from build123d import *

# Parameters (mm, degrees)
SKETCH1_R           = 4
BOSS_EXTRUDE1_DEPTH = 5
BOSS_EXTRUDE1_TAPER = 13
SKETCH2_R           = 4
BOSS_EXTRUDE2_DEPTH = 5
BOSS_EXTRUDE2_TAPER = 13
SKETCH3_R           = 4
BOSS_EXTRUDE3_DEPTH = 5
BOSS_EXTRUDE3_TAPER = 13
SKETCH4_R           = 2.85
BOSS_EXTRUDE4_DEPTH = 2
SKETCH5_R           = 2.85
BOSS_EXTRUDE5_DEPTH = 3
BOSS_EXTRUDE5_DRAFT = -35
SKETCH6_R           = 4.950622615
BOSS_EXTRUDE6_DEPTH = 15
BOSS_EXTRUDE6_TAPER = 12
SKETCH9_R           = 2
CUT_EXTRUDE1_DEPTH  = 20


with BuildPart() as part:
    # Sketch1 → Boss-Extrude1 (new body)
    with BuildSketch(Plane(origin=(0, 0, 0), x_dir=(0, 0, -1), z_dir=(1, 0, 0))):
        Circle(SKETCH1_R)
    extrude(amount=BOSS_EXTRUDE1_DEPTH, taper=BOSS_EXTRUDE1_TAPER)

    # Sketch2 → Boss-Extrude2 (add)
    with BuildSketch(Plane(origin=(5, 0, 0), x_dir=(0, 0, -1), z_dir=(1, 0, 0))):
        Circle(SKETCH2_R)
    extrude(amount=BOSS_EXTRUDE2_DEPTH, taper=BOSS_EXTRUDE2_TAPER)

    # Sketch3 → Boss-Extrude3 (add)
    with BuildSketch(Plane(origin=(10, 0, 0), x_dir=(0, 0, -1), z_dir=(1, 0, 0))):
        Circle(SKETCH3_R)
    extrude(amount=BOSS_EXTRUDE3_DEPTH, taper=BOSS_EXTRUDE3_TAPER)

    # Sketch4 → Boss-Extrude4 (add)
    with BuildSketch(Plane.ZY):
        Circle(SKETCH4_R)
    extrude(amount=BOSS_EXTRUDE4_DEPTH)


with BuildPart() as boss_extrude5_tool:
    # Sketch5 → Boss-Extrude5 (with draft: the straight prism first)
    with BuildSketch(Plane.ZY.offset(2)):
        Circle(SKETCH5_R)
    extrude(amount=BOSS_EXTRUDE5_DEPTH)
    # Boss-Extrude5: the draft: its side faces are tilted about the plane it starts from
    boss_extrude5_sides = [boss_extrude5_tool.faces().sort_by_distance(p)[0] for p in [
        (-3.5, 0, -2.85),
    ]]
    draft(boss_extrude5_sides, Plane.ZY.offset(2), BOSS_EXTRUDE5_DRAFT)


with BuildPart() as part_1:
    add(part.part)

    # Boss-Extrude5: add boss_extrude5_tool
    add(boss_extrude5_tool.part)

    # Sketch6 → Boss-Extrude6 (add)
    with BuildSketch(Plane.ZY.offset(5)):
        Circle(SKETCH6_R)
    extrude(amount=BOSS_EXTRUDE6_DEPTH, taper=BOSS_EXTRUDE6_TAPER)

    # Sketch9 → Cut-Extrude1 (cut)
    with BuildSketch(Plane(origin=(15, 0, 0), x_dir=(0, 0, -1), z_dir=(1, 0, 0))):
        Circle(SKETCH9_R)
    extrude(amount=-CUT_EXTRUDE1_DEPTH, mode=Mode.SUBTRACT)


solid = part_1.part
Could you check a few things on this model? Use its own coordinates, in mm. A direction names the side the tool comes from. Give positions to 0.01 mm unless a question says otherwise; leave off trailing zeros. Order: outer loops, then holes, each group sorted by start corner. A loop starts at its lowest first (then second) coordinate and runs counter-clockwise, first axis right, second up.
Item 1: If we section it at B-B, the plane x = 1: Write out the boundary of the cut face in (y, z), plus the area to 3 significant figures.
Item 2: For faces 1 (the face through (-0.986, -1.734, -2.262)), 2 (the face through (-20, 0, 0)), 3 (the face through (-5, 0, 0)), which set-ups out of +Z, -Z, +X, -X, +Y, -Y let a thin tool reach every point of the face, with its end or its side?
Item 3: If we section it at A-A, the plane z = 0: Write out the boundary of the cut face in (x, y), plus the area to 3 significant figures.
Item 4: If we section it at C-C, the plane x = -10.5: Write out the boundary of the cut face in (y, z).
Item 5: I need wall thicknesses on line 1 (Z direction, x = -1, y = -1); line 2 (X direction, y = -1.5, z = -0.25); line 3 (Y direction, x = 1.75, z = 0). Which ranges of each line are inside material? Lowest first, please.
Item 6: If we mould it in two halves opening along X, with no side actions, what happens to faces 4 (the face through (5, 3, -1)), 5 (the face through (-12.605, -3.255, -0.723)), 6 (the face through (5, -2, 0))? For each: pulls with the +X half, pulls with the -X half, needs draft (parallel to the pull), parting line crosses it, or undercut.
Item 7: If we section it at D-D, the plane x = -3.5: Write out the boundary of the cut face in (y, z).
Item 8: I'm going to push flat-ended pins straight in: pin 1 (1 mm diameter, centred on x = 8.5, z = -0.5, fed in from -Y); pin 2 (1 mm diameter, centred on x = -7, y = -3, fed in from -Z); pin 3 (3.5 mm diameter, centred on y = 0, z = 0, fed in from +X). Where does each tip first touch, or does it pass through?
Values:
1. outline: circle Ø7.54 at (0, 0); hole circle Ø4 at (0, 0)
1. area: 32.1 mm2
2. face 1: none
2. face 2: +Z, -Z, -X, +Y, -Y
2. face 3: +X
3. outline: (-20, -1.76) - (-5, -4.95) - (-2, -2.85) - (0, -2.85) - (0, -4) - (5, -2.85) - (5, -4) - (10, -2.85) - (10, -4) - (15, -2.85) - (15, -2) - (-5, -2) - (-5, 2) - (15, 2) - (15, 2.85) - (10, 4) - (10, 2.85) - (5, 4) - (5, 2.85) - (0, 4) - (0, 2.85) - (-2, 2.85) - (-5, 4.95) - (-20, 1.76) - close
3. area: 158 mm2
4. outline: circle Ø7.56 at (0, 0)
5. line 1: z = -2.67 to -1.73, 1.73 to 2.67
5. line 2: x = -20 to -5
5. line 3: y = -3.6 to -2, 2 to 3.6
6. face 4: undercut
6. face 5: pulls with the -X half
6. face 6: needs draft
7. outline: circle Ø7.8 at (0, 0); hole circle Ø4 at (0, 0)
8. pin 1: stops at y = -3.28
8. pin 2: stops at z = -3.8
8. pin 3: stops at x = -5
